```python
from build123d import *

# Parameters (mm, degrees)
F2_SIZE = 1
F3_SIZE = 0.5


with BuildPart() as f1:
    # F0 (on Front) → F1 (revolve)
    with BuildSketch(Plane.XZ):
        Polygon((15.4, 10.5), (0, 10.5), (0, 12.675), (-2.5, 12.675), (-2.5, 7.55), (15.4, 7.55), align=None)
    revolve(axis=Axis((7.2899, 0, 0), (1, 0, 0)))

    # F2
    f2_edges = [f1.edges().sort_by_distance(p)[0] for p in [
        (15.4, 0, -10.5),
    ]]
    chamfer(f2_edges, length=F2_SIZE)

    # F3
    f3_edges = [f1.edges().sort_by_distance(p)[0] for p in [
        (-2.5, 0, -12.675),
        (-2.5, 0, -7.55),
        (15.4, 0, -7.55),
    ]]
    chamfer(f3_edges, length=F3_SIZE)


solid = f1.part
```
Verification items for the finished model (mm, model axes). A direction names the side the tool comes from. Give positions to 0.01 mm unless a question says otherwise; leave off trailing zeros. Order: outer loops, then holes, each group sorted by start corner. A loop starts at its lowest first (then second) coordinate and runs counter-clockwise, first axis right, second up. Notation, with made-up numbers: (83, 8.5) -> (97, 8.5) arc R21 ccw to (97, 24.5) -> close; hole circle Ø1 at (67.5, 27). An arc over 180 degrees is marked (long way). Use a Markdown table: item, result.
1) Section check A-A, the plane z = 0. Record the boundary of the cut face in (x, y) (3 decimals).
Results:
| item | result |
|---|---|
| outline | (-2.5, -12.175) -> (-2, -12.675) -> (0, -12.675) -> (0, -10.5) -> (14.4, -10.5) -> (15.4, -9.5) -> (15.4, -8.05) -> (14.9, -7.55) -> (-2, -7.55) -> (-2.5, -8.05) -> close; (-2.5, 8.05) -> (-2, 7.55) -> (14.9, 7.55) -> (15.4, 8.05) -> (15.4, 9.5) -> (14.4, 10.5) -> (0, 10.5) -> (0, 12.675) -> (-2, 12.675) -> (-2.5, 12.175) -> close |
2) Section check C-C, the plane x = 2.25. Record the boundary of the cut face in (y, z).
Results:
| item | result |
|---|---|
| outline | circle Ø21 at (0, 0); hole circle Ø15.1 at (0, 0) |
3) Tool access check on faces 4 (the flat face through (15.4, -2, 8)), 5 (the cylindrical face through (7.1, -3.2, 10)). Record the directions out of +Z, -Z, +X, -X, +Y, -Y that give a thin tool (end or side, any length) a straight path to the whole face; none if there is none.
Results:
| item | result |
|---|---|
| face 4 | +Z, -Z, +X, +Y, -Y |
| face 5 | +X |
4) Material ranges on probe 1 along Y at (x, z) = (2, 0); probe 2 along Z at (x, y) = (3.5, -6.5), recorded low to high.
Results:
| item | result |
|---|---|
| probe 1 | -10.5 to -7.55, 7.55 to 10.5 |
| probe 2 | -8.25 to -3.84, 3.84 to 8.25 |
5) Mould release check, pull along Z, two halves, no side actions. Record for faces 1 (the cylindrical face through (-1.01, -3.81, 12.09)), 2 (the cylindrical face through (6.57, 7.37, -1.64)), 3 (the flat face through (0, -8, 8)): pulls with the +Z half, pulls with the -Z half, needs draft (parallel to the pull), parting line crosses it, or undercut.
Results:
| item | result |
|---|---|
| face 1 | parting line crosses it |
| face 2 | undercut |
| face 3 | needs draft |
6) Depth check by flat-ended pin: pin 1 Ø2 at (y, z) = (3, -10) entering from +X; pin 2 Ø1.5 at (y, z) = (-9.5, -7) entering from +X; pin 3 Ø4 at (x, z) = (3.5, 7) entering from +Y; pin 4 Ø3 at (x, z) = (12, -3) entering from -Y. Enter the tip coordinate at first touch or a pass-through.
Results:
| item | result |
|---|---|
| pin 1 | x = 15.4 |
| pin 2 | x = 0 |
| pin 3 | y = 9.23 |
| pin 4 | y = -10.39 |
